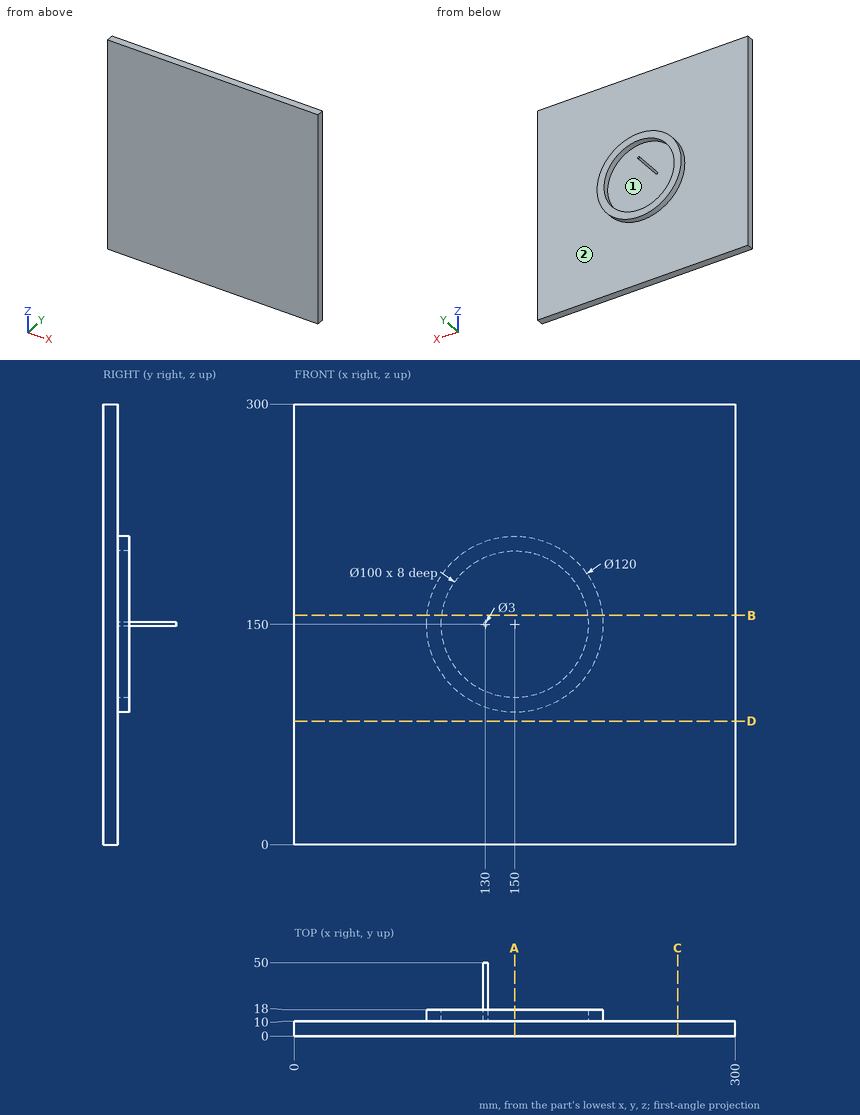
Job drawing, mm, ordinate dimensions from the low corner. One solid piece. Coordinates: 2 decimals unless noted, no trailing zeros. Loops run counter-clockwise (first coordinate to the right, second up) from the corner with the lowest first, then second, coordinate; pieces in that order, holes last. Notation, with made-up numbers: (6.25, 28) - (48.25, 28) arc R18 ccw to (48.25, 56) - close; hole circle Ø4 at (15.5, 28). An arc over 180 degrees is marked (long way). Answer as a JSON object with one key per item and string values. Group by question number.
(1) Flat gauge pins, fed straight in: pin 1 (4 mm diameter, centred on x = 247.5, z = 136.5, fed in from +Y); pin 2 (10 mm diameter, centred on y = 11.5, z = 184, fed in from +X); pin 3 (1.5 mm diameter, centred on y = 19, z = 169.5, fed in from -X). Where does each tip first touch, or does it go through?
(2) Cut at D-D (z = 84). Give the cut face in (x, y), then the cut area to 3 significant figures.
(3) Cut at B-B (z = 156). Give the cut face in (x, y).
(4) Cut at C-C (x = 261). Give the cut face in (y, z), then the cut area to 3 significant figures.
(5) Probe line 1 along X through (y, z) = (13, 150); line 2 along Z through (x, y) = (150, 13); line 3 along Y through (x, z) = (123, 238). List the from-to ranges inside material, lowest first.
(6) Two-plate mould, pull along Z, no slides. Class the marked faces 1 and 2: released by +Z, released by -Z, zero draft, split by the parting line, or undercut.
(7) Cut at A-A (x = 150). Give the cut face in (y, z), then the cut area to 3 significant figures.
Geometry says:
{
 "1": {"pin 1": "stops at y = 10", "pin 2": "stops at x = 300", "pin 3": "passes through"},
 "2": {"outline": "(0, 0) - (300, 0) - (300, 10) - (0, 10) - close", "area": "3,000 mm^2"},
 "3": {"outline": "(0, 0) - (300, 0) - (300, 10) - (209.7, 10) - (209.7, 18) - (199.64, 18) - (199.64, 10) - (100.36, 10) - (100.36, 18) - (90.3, 18) - (90.3, 10) - (0, 10) - close"},
 "4": {"outline": "(0, 0) - (10, 0) - (10, 300) - (0, 300) - close", "area": "3,000 mm^2"},
 "5": {"line 1": "x = 90 to 100, 128.5 to 131.5, 200 to 210", "line 2": "z = 90 to 100, 200 to 210", "line 3": "y = 0 to 10"},
 "6": {"face 1": "undercut", "face 2": "zero draft"},
 "7": {"outline": "(0, 0) - (10, 0) - (10, 90) - (18, 90) - (18, 100) - (10, 100) - (10, 200) - (18, 200) - (18, 210) - (10, 210) - (10, 300) - (0, 300) - close", "area": "3,160 mm^2"}
}
